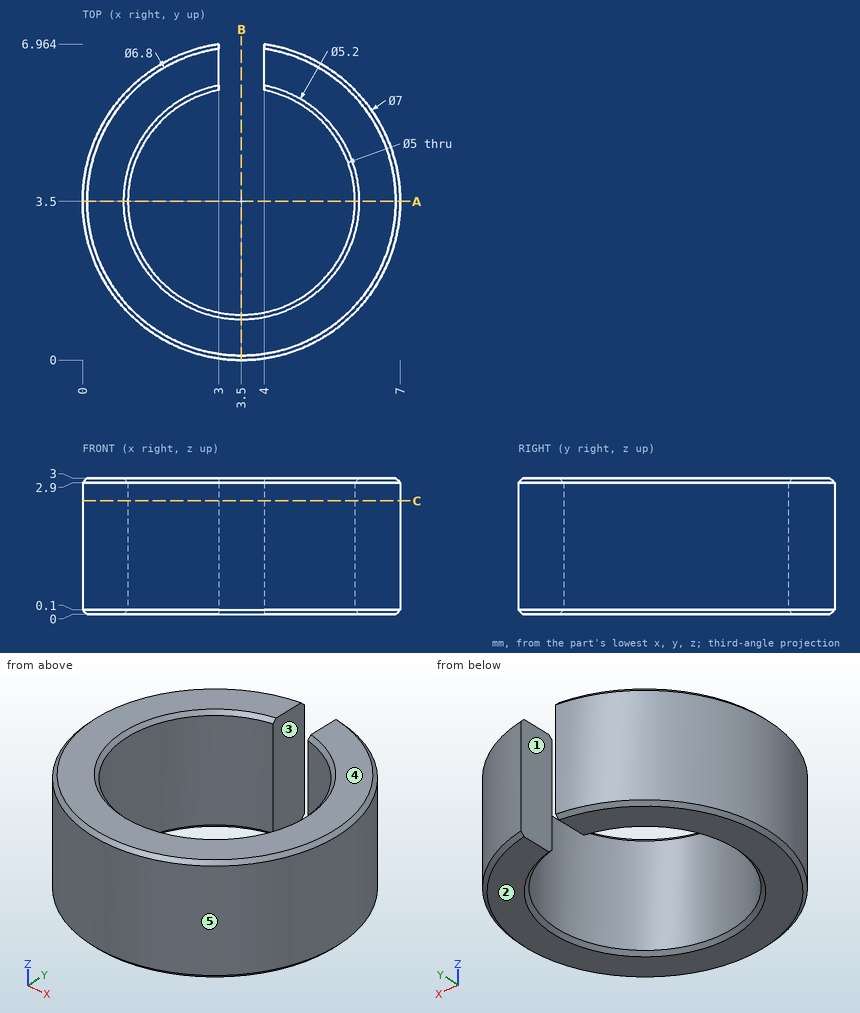
Job drawing, mm, ordinate dimensions from the low corner. One solid piece. A direction names the side the tool comes from. Round coordinates to 2 decimals unless told otherwise and drop trailing zeros. Order: outer loops, then holes, each group sorted by start corner. A loop starts at its lowest first (then second) coordinate and runs counter-clockwise, first axis right, second up. Notation, with made-up numbers: (3, -35.5) - (22, -35.5) arc R30 ccw to (22, -7.5) - close; hole circle Ø4 at (62.5, 3). An arc over 180 degrees is marked (long way). Use CSV: the item, a comma, the result in double quotes. Start each with the question number.
1) Saw through at B-B (x = 3.5). List the corners of the cut face in (y, z).
2) Two-plate mould, pull along X, no slides. Class the marked faces 3, 4 and 5: pulls with the +X half, pulls with the -X half, needs draft (parallel to the pull), parting line crosses it, or undercut.
3) Saw through at A-A (y = 3.5). List the corners of the cut face in (x, z).
4) Wall check: L1, parallel to X at y = 3.5, z = 1.5; L2, parallel to Y at x = 3.5, z = 1.8; L3, parallel to X at y = 5.75, z = 1.7. Give the ranges that are in metal, low to high. Write a range as [from, to].
5) Saw through at C-C (z = 2.5). List the corners of the cut face in (x, y).
6) Pin check, flat tips, straight feed: pin 1 Ø1.1 at (y, z) = (6.5, 1) entering from -X; pin 2 Ø1.1 at (y, z) = (6.5, 2) entering from +X. Stop position of each tip, or through.
7) Tool access for the marked faces 1 and 2: list every direction of +Z, -Z, +X, -X, +Y, -Y with a clear straight run to the whole face (end or side of a thin tool).
Values follow:
1,outline,"(0, 0.1) - (0.1, 0) - (0.9, 0) - (1, 0.1) - (1, 2.9) - (0.9, 3) - (0.1, 3) - (0, 2.9) - close"
2,face 3,"undercut"
2,face 4,"needs draft"
2,face 5,"parting line crosses it"
3,outline,"(0, 0.1) - (0.1, 0) - (0.9, 0) - (1, 0.1) - (1, 2.9) - (0.9, 3) - (0.1, 3) - (0, 2.9) - close; (6, 0.1) - (6.1, 0) - (6.9, 0) - (7, 0.1) - (7, 2.9) - (6.9, 3) - (6.1, 3) - (6, 2.9) - close"
4,L1,"x = [0, 1], [6, 7]"
4,L2,"y = [0, 1]"
4,L3,"x = [0.82, 2.41], [4.59, 6.18]"
5,outline,"(3, 5.95) - (3, 6.96) arc R3.5 ccw (long way) to (4, 6.96) - (4, 5.95) arc R2.5 cw (long way) to start"
6,pin 1,"stops at x = 1"
6,pin 2,"stops at x = 6"
7,face 1,"+Z, -Z, +Y"
7,face 2,"-Z, +X, -X, +Y, -Y"
